from build123d import *

# Parameters (mm, degrees)
F2_SIZE2 = 1.524
F2_SIZE  = 1.524


with BuildPart() as f1:
    # F0 (on Right) → F1 (revolve)
    with BuildSketch(Plane.YZ):
        with BuildLine():
            Line((-11.1125, 6.35), (-11.1125, 0))
            Line((-11.1125, 0), (0, 0))
            Line((0, 0), (0, 26.9748))
            Line((0, 26.9748), (-3.175, 26.9748))
            Line((-3.175, 26.9748), (-3.175, 12.7))
            Line((-3.175, 12.7), (-7.9375, 12.7))
            ThreePointArc((-7.9375, 12.7), (-8.774141, 9.14957), (-11.1125, 6.35))
        make_face()
    revolve(axis=Axis((0, 0, 13.4874), (0, 0, 1)))

    # F2
    f2_edges = [f1.edges().sort_by_distance(p)[0] for p in [
        (0, 11.1125, 0),
    ]]
    chamfer(f2_edges, length=F2_SIZE, length2=F2_SIZE2)


solid = f1.part
Check sheet for the modelled part. Datum: model origin and axes. Units: mm. A direction names the side the tool comes from. Round coordinates to 2 decimals unless told otherwise and drop trailing zeros. Loops run counter-clockwise (first coordinate to the right, second up) from the corner with the lowest first, then second, coordinate; pieces in that order, holes last. Notation, with made-up numbers: M 54.25,-32.5 L 98.25,-32.5 A29 cw 98.25,5.5 Z; hole C 48,4 d11. An arc over 180 degrees is marked long. One line per question, with ' | ' between items. Start each with the question number.
Item 1: Gauge pin test, flat ends, axial feed: pin 1 Ø4 at (y, z) = (1.5, 10) entering from -X; pin 2 Ø1 at (x, z) = (-6, 3) entering from +Y; pin 3 Ø5 at (x, z) = (-8, 10.5) entering from -Y; pin 4 Ø10 at (x, y) = (6.5, -1) entering from +Z. Record the tip position at first contact, or that the pin passes through.
Item 2: Section check C-C (z = 4.5). Record the boundary of the cut face in (x, y) (1 decimal), and give its area (3 significant figures).
Item 3: Scan lines: probe 1 along Z at (x, y) = (-6, -1.75); probe 2 along Y at (x, z) = (2.75, 15); probe 3 along Y at (x, z) = (-9, 2.25). Record each from-to range of solid material in increasing order.
Item 4: Set-up check for faces 1 (the face through (0, 0, 26.975)), 2 (the face through (0.1, 3.4, 12.7)): record each of +Z, -Z, +X, -X, +Y, -Y from which the full face is reachable in a straight line by a thin tool's end or side.
Item 5: Section check D-D (z = 11). Record the boundary of the cut face in (x, y).
Worked out:
1) pin 1: x = -9.38 | pin 2: y = 9.66 | pin 3: y = -6.51 | pin 4: z = 26.97
2) outline: C 0,0 d22.2 | area: 388 mm^2
3) probe 1: 0 to 12.7 | probe 2: -1.59 to 1.59 | probe 3: -6.52 to 6.52
4) face 1: +Z, +X, -X, +Y, -Y | face 2: +Z
5) outline: C 0,0 d16.24
